Source: CAD feature listing. Evaluate the final solid. Frame: model axes, mm. Face numbers are marked on the shaded views. A direction names the side the tool comes from. Round coordinates to 2 decimals unless told otherwise and drop trailing zeros. Write each loop counter-clockwise with the first axis right and the second up, starting at its lowest first coordinate (ties: lowest second). Pieces come first, ordered by that corner, then holes.
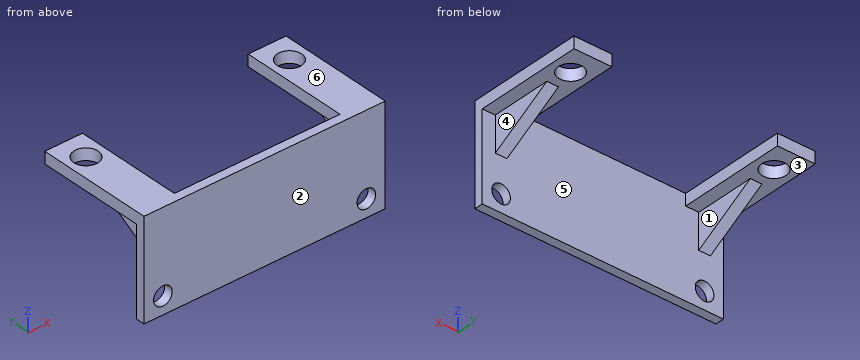
Autodesk Inventor part; units mm, degrees
ref_plane "XZ Plane" through (0, 0, 0) normal (0, 1, 0) x (-1, 0, 0)
ref_plane "XY Plane" through (0, 0, 0) normal (0, 0, 1) x (1, 0, 0)
sketch "スケッチ1" plane through (0, 0, 0) normal (0, 0, 1) x (1, 0, 0)
  line L0 (0, 0) -> (0, 23.3181) construction
  line L1 (-22.6457, 15.5) -> (22.6457, 15.5) construction
  line L2 (-20.3832, 1.5) -> (20.3832, 1.5) construction
  circle A0 centre (0, 15.5) radius 14 construction
  line L3 (-22.6457, 7.5) -> (22.6457, 7.5) construction
  circle A1 centre (-17.5, 15.5) radius 2.1
  circle A2 centre (17.5, 15.5) radius 2.1
  line L4 (-14.25, 20) -> (-20.75, 20)
  line L5 (-20.75, 20) -> (-20.75, 0)
  line L6 (-20.75, 0) -> (-14.25, 0)
  line L7 (-14.25, 0) -> (-14.25, 20)
  line L8 (14.25, 20) -> (20.75, 20)
  line L9 (20.75, 20) -> (20.75, 0)
  line L10 (20.75, 0) -> (14.25, 0)
  line L11 (14.25, 0) -> (14.25, 20)
  line L12 (20.75, 0) -> (20.75, 1.5)
  line L13 (20.75, 1.5) -> (-20.75, 1.5)
  line L14 (-20.75, 1.5) -> (-20.75, 0)
  line L15 (-20.75, 0) -> (20.75, 0)
  point P0 (0, 1.5)
  point P1 (0, 7.5)
  point P2 (-17.5, 20)
  point P3 (17.5, 20)
  point P4 (-14.25, 0)
  point P5 (14.25, 0)
  point P6 (14.25, 1.5)
  point P7 (-14.25, 1.5)
  point P8 (-20.75, 1.5)
  dimension "d0" = 28
  dimension "d1" = 1.5
  dimension "d2" = 8
  dimension "d3" = 4.2
  dimension "d4" = 35
  dimension "d5" = 6.5
  dimension "d6" = 20
extrude "前" add sketch "スケッチ1" along normal blind 2
extrude "底" add sketch "スケッチ1" against normal blind 15 contours L13 L11 L15 L7 | L7 L6 L5 L13 | L13 L9 L10 L11
ref_plane "作業平面1" through (17.5, 0, 0) normal (1, 0, 0) x (0, 1, 0)
sketch "スケッチ2" plane through (17.5, 0, 0) normal (1, 0, 0) x (0, 1, 0)
  line L0 (11.8923, 0) -> (1.5, -6)
  line L1 (1.5, 0) -> (1.5, -15)
  line L2 (1.5, 0) -> (20, 0)
  line L3 (11.8923, 0) -> (1.5, 0)
  line L4 (1.5, 0) -> (1.5, -6)
  point P0 (0, 0)
  dimension "d12" = 60
  dimension "d13" = 6
extrude "リブ" add sketch "スケッチ2" along normal mid plane 2
mirror "ミラー1" about plane through (0, 0, 0) normal (1, 0, 0) of "リブ"
sketch "スケッチ3" plane through (-14.25, 1.5, 2) normal (0, 1, 0) x (1, 0, 0)
  line L0 (14.25, -18.7393) -> (14.25, 26.1406) construction
  line L1 (41.5884, 14) -> (-17.6431, 14) construction
  line L2 (35, 0) -> (28.5, 0) construction
  point P0 (14.25, 2)
  point P1 (31.75, 14)
  point P2 (-3.25, 14)
  dimension "d16" = 35
  dimension "d17" = 14
hole "穴1" at (17.5, 1.5, -12) at (-17.5, 1.5, -12) direction (0, -1, 0) diameter 3.2 end through all
properties part number "28BYJ-48_Braket"
Q1. Section query C-C, the plane y = 3. Output: boundary loops of the cut face in (x, z).
Q2. Section query A-A, the plane y = 15.5. Output: boundary loops of the cut face in (x, z), and give its area (3 significant figures).
Q3. Section query B-B, the plane x = -17.5. Output: boundary loops of the cut face in (y, z).
Q4. Line query: line 1 (X direction, y = 0.45, z = -12); line 2 (Z direction, x = -17.5, y = 0.85); line 3 (X direction, y = 2, z = -1). Output: solid intervals per line, ascending.
Q5. Section query D-D, the plane z = -5.5. Output: boundary loops of the cut face in (x, y).
Q6. Set-up query: the marked faces 1 and 2. Return all of +Z, -Z, +X, -X, +Y, -Y with unobstructed straight access to the full face (end or side cutting, diameter ignored); none if empty.
Q7. Mould query, pull axis X, two halves, no side actions, for the marked faces 3, 4, 5 and 6. Classes: pulls with the +X half, pulls with the -X half, needs draft (parallel to the pull), parting line crosses it, or undercut.
Q8. Pin query (flat end, axial travel): P1, Ø5, axis at y = 13, z = -4.5, coming from the +X side; P2, Ø5, axis at x = -3, z = -11.5, coming from the +Y side; P3, Ø6.5, axis at y = 7, z = -3.5, coming from the -X side; P4, Ø2, axis at x = 16, y = 12, coming from the -Z side. Return the tip coordinate at first contact, or that it passes through.
Filled in:
1. outline: (-20.75, 0) - (-18.5, 0) - (-18.5, -5.13) - (-16.5, -5.13) - (-16.5, 0) - (-14.25, 0) - (-14.25, 2) - (-20.75, 2) - close; (14.25, 0) - (16.5, 0) - (16.5, -5.13) - (18.5, -5.13) - (18.5, 0) - (20.75, 0) - (20.75, 2) - (14.25, 2) - close
2. outline: (-20.75, 0) - (-19.6, 0) - (-19.6, 2) - (-20.75, 2) - close; (-15.4, 0) - (-14.25, 0) - (-14.25, 2) - (-15.4, 2) - close; (14.25, 0) - (15.4, 0) - (15.4, 2) - (14.25, 2) - close; (19.6, 0) - (20.75, 0) - (20.75, 2) - (19.6, 2) - close
2. area: 9.20 mm2
3. outline: (0, -15) - (1.5, -15) - (1.5, -13.6) - (0, -13.6) - close; (0, -10.4) - (1.5, -10.4) - (1.5, -6) - (11.89, 0) - (13.4, 0) - (13.4, 2) - (0, 2) - close; (17.6, 0) - (20, 0) - (20, 2) - (17.6, 2) - close
4. line 1: x = -20.75 to -19.1, -15.9 to 15.9, 19.1 to 20.75
4. line 2: z = -15 to -13.6, -10.4 to 2
4. line 3: x = -18.5 to -16.5, 16.5 to 18.5
5. outline: (-20.75, 0) - (20.75, 0) - (20.75, 1.5) - (18.5, 1.5) - (18.5, 2.37) - (16.5, 2.37) - (16.5, 1.5) - (-16.5, 1.5) - (-16.5, 2.37) - (-18.5, 2.37) - (-18.5, 1.5) - (-20.75, 1.5) - close
6. face 1: -Z, +Y
6. face 2: +Z, -Z, +X, -X, -Y
7. face 3: undercut
7. face 4: pulls with the +X half
7. face 5: undercut
7. face 6: needs draft
8. P1: passes through
8. P2: stops at y = 1.5
8. P3: stops at x = -18.5
8. P4: stops at z = -0.44
